from build123d import *

# Parameters (mm, degrees)
CROQUIS1_R              = 50
CROQUIS1_R_2            = 19
SALIENTE_EXTRUIR1_DEPTH = 5
CROQUIS4_R              = 30
CROQUIS4_R_2            = 20.75
CORTAR_EXTRUIR1_DEPTH   = 2
CROQUIS5_R              = 2.75
CORTAR_EXTRUIR2_DEPTH   = 5


with BuildPart() as part:
    # Croquis1 → Saliente-Extruir1 (new body)
    with BuildSketch(Plane.XY):
        Circle(CROQUIS1_R)
        Circle(CROQUIS1_R_2, mode=Mode.SUBTRACT)
    extrude(amount=SALIENTE_EXTRUIR1_DEPTH)

    # Croquis4 → Cortar-Extruir1 (cut)
    with BuildSketch(Plane.XY.offset(5)):
        Circle(CROQUIS4_R)
        Circle(CROQUIS4_R_2, mode=Mode.SUBTRACT)
    extrude(amount=-CORTAR_EXTRUIR1_DEPTH, mode=Mode.SUBTRACT)

    # Croquis5 → Cortar-Extruir2 (cut)
    with BuildSketch(Plane.XY.offset(5)):
        with Locations((40.602997929, 0)):
            Circle(CROQUIS5_R)
        with Locations((28.710655172, -28.710655172)):
            Circle(CROQUIS5_R)
        with Locations((0, -40.602997929)):
            Circle(CROQUIS5_R)
        with Locations((-28.710655172, -28.710655172)):
            Circle(CROQUIS5_R)
        with Locations((-40.602997929, 0)):
            Circle(CROQUIS5_R)
        with Locations((-28.710655172, 28.710655172)):
            Circle(CROQUIS5_R)
        with Locations((0, 40.602997929)):
            Circle(CROQUIS5_R)
        with Locations((28.710655172, 28.710655172)):
            Circle(CROQUIS5_R)
    extrude(amount=-CORTAR_EXTRUIR2_DEPTH, mode=Mode.SUBTRACT)


solid = part.part
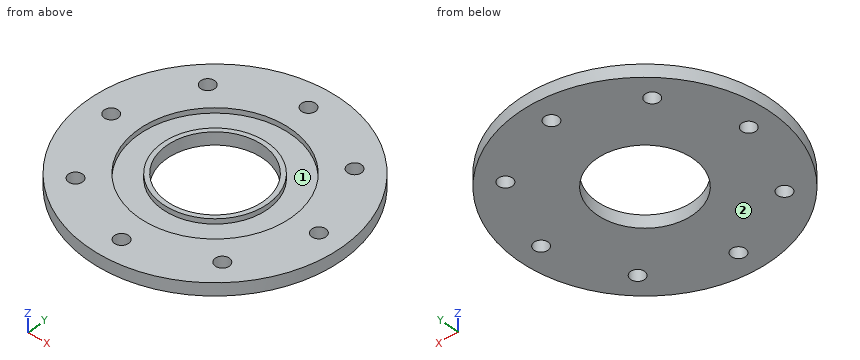
Geometry: final body of the model. Coordinates: model frame, mm. Face numbers are marked on the shaded views. Give positions to 0.01 mm unless a question says otherwise; leave off trailing zeros. Loops run counter-clockwise (first coordinate to the right, second up) from the corner with the lowest first, then second, coordinate; pieces in that order, holes last. Notation, with made-up numbers: M -12,27 L 23,27 A17 cw 23,41 Z; hole C -25,26 d5. An arc over 180 degrees is marked long. Put each result on its own line as item: value.
1) Cut plane C-C, the plane y = -11. Return the cut outline in (x, z) (3 decimals), plus the area to 3 significant figures.
Computed values:
outline: M -48.775,0 L -15.492,0 L -15.492,5 L -17.594,5 L -17.594,3 L -27.911,3 L -27.911,5 L -48.775,5 Z; M 15.492,0 L 48.775,0 L 48.775,5 L 27.911,5 L 27.911,3 L 17.594,3 L 17.594,5 L 15.492,5 Z
area: 292 mm^2
2) Cut plane A-A, the plane x = 0. Return the cut outline in (y, z), plus the area to 3 significant figures.
Computed values:
outline: M -50,0 L -43.35,0 L -43.35,5 L -50,5 Z; M -37.85,0 L -19,0 L -19,5 L -20.75,5 L -20.75,3 L -30,3 L -30,5 L -37.85,5 Z; M 19,0 L 37.85,0 L 37.85,5 L 30,5 L 30,3 L 20.75,3 L 20.75,5 L 19,5 Z; M 43.35,0 L 50,0 L 50,5 L 43.35,5 Z
area: 218 mm^2
3) Cut plane D-D, the plane x = 13.5. Return the cut outline in (y, z).
Computed values:
outline: M -48.14,0 L -13.37,0 L -13.37,5 L -15.76,5 L -15.76,3 L -26.79,3 L -26.79,5 L -48.14,5 Z; M 13.37,0 L 48.14,0 L 48.14,5 L 26.79,5 L 26.79,3 L 15.76,3 L 15.76,5 L 13.37,5 Z
4) Material intervals for L1, parallel to Y at x = 0, z = 2.3; L2, parallel to X at y = 2, z = 2.75; L3, parallel to X at y = -2.5, z = 4.65, sorted ascending. Write a range as from..to.
Computed values:
L1: y = -50..-43.35, -37.85..-19, 19..37.85, 43.35..50
L2: x = -49.96..-42.49, -38.72..-18.89, 18.89..38.72, 42.49..49.96
L3: x = -49.94..-41.75, -39.46..-29.9, -20.6..-18.83, 18.83..20.6, 29.9..39.46, 41.75..49.94
5) Mould query, pull axis Y, two halves, no side actions, for the marked faces 1 and 2. Classes: released by +Y, released by -Y, zero draft, split by the parting line, or undercut.
Computed values:
face 1: undercut
face 2: zero draft
6) First-contact query: P1, Ø2, axis at y = -2.5, z = 2.5, coming from the -X side; P2, Ø1.5, axis at x = 18.5, y = -19.5, coming from the +Z side; P3, Ø1.5, axis at y = 22.5, z = 0.5, coming from the +X side; P4, Ø5, axis at x = 0, y = -40.6, coming from the +Z side. Flat tips, straight axial feed; report the tip coordinate or a pass-through.
Computed values:
P1: stops at x = -49.98
P2: stops at z = 3
P3: stops at x = 45.02
P4: passes through
